from build123d import *

# Parameters (mm, degrees)
SKETCH_1_W          = 226
SKETCH_1_H          = 45
EXTRUDE_1_DEPTH     = 1
SKETCH_2_R          = 1.65
CUT_EXTRUDE_1_DEPTH = 116.222610628
CUT_EXTRUDE_2_DEPTH = 10
SKETCH_4_R          = 1.65
CUT_EXTRUDE_3_DEPTH = 116.222610628


with BuildPart() as part:
    # 草图1 → 凸台-拉伸1 (new body)
    with BuildSketch(Plane.XY):
        Rectangle(SKETCH_1_W, SKETCH_1_H)
    extrude(amount=EXTRUDE_1_DEPTH)

    # 草图2 → 切除-拉伸1 (cut, through all)
    with BuildSketch(Plane.XY.offset(1)):
        with Locations((90, 19.5)):
            Circle(SKETCH_2_R)
        with Locations((70, 19.5)):
            Circle(SKETCH_2_R)
        with Locations(Location((-70, 19.5, 0), (0, 0, 180))):
            Circle(SKETCH_2_R)
        with Locations(Location((-90, 19.5, 0), (0, 0, 180))):
            Circle(SKETCH_2_R)
    extrude(amount=-CUT_EXTRUDE_1_DEPTH, mode=Mode.SUBTRACT)

    # 草图3 → 切除-拉伸2 (cut)
    with BuildSketch(Plane.XY.offset(1)):
        with BuildLine():
            Line((-80, 6), (80, 6))
            ThreePointArc((80, 6), (86, 0), (80, -6))
            Line((80, -6), (-80, -6))
            ThreePointArc((-80, -6), (-86, 0), (-80, 6))
        make_face()
    extrude(amount=-CUT_EXTRUDE_2_DEPTH, mode=Mode.SUBTRACT)

    # 草图4 → 切除-拉伸3 (cut, through all)
    with BuildSketch(Plane.XY.offset(1)):
        with Locations((109, 7.5)):
            Circle(SKETCH_4_R)
        with Locations((109, -12.5)):
            Circle(SKETCH_4_R)
        with Locations(Location((-109, -12.5, 0), (0, 0, 180))):
            Circle(SKETCH_4_R)
        with Locations(Location((-109, 7.5, 0), (0, 0, 180))):
            Circle(SKETCH_4_R)
    extrude(amount=-CUT_EXTRUDE_3_DEPTH, mode=Mode.SUBTRACT)


solid = part.part
Could you check a few things on this model? Use its own coordinates, in mm. A direction names the side the tool comes from. Round coordinates to 2 decimals unless told otherwise and drop trailing zeros. Write each loop counter-clockwise with the first axis right and the second up, starting at its lowest first coordinate (ties: lowest second). Pieces come first, ordered by that corner, then holes. Notation, with made-up numbers: (-40, 9) - (7, 9) arc R21 ccw to (7, 34) - close; hole circle Ø8 at (10.25, -35). An arc over 180 degrees is marked (long way). Put each result on its own line as item: value. Start each with the question number.
(1) Thinking about a two-plate mould opening in Y: for faces 1 (the cylindrical face through (86, 0.1, 0.5)), 2 (the flat face through (-2, 10, 0)), which applies, released by +Y, released by -Y, zero draft, split by the parting line, or undercut?
(2) I want a section at B-B, the plane z = 0.5. Give the number of separate pieces and of enclosed holes in the cut face, plus the area to 3 significant figures.
(3) I need wall thicknesses on probe 1 along Y at (x, z) = (90, 0.7); probe 2 along X at (y, z) = (0, 0.95); probe 3 along Y at (x, z) = (45, 0.25). Which ranges of each line are inside material? Lowest first, please.
(4) I want a section at A-A, the plane y = 0. Please give me the cut outline in (x, z).
(5) For faces 3 (the flat face through (-2, 10, 1)), 4 (the cylindrical face through (-86, -0.1, 0.5)), which set-ups out of +Z, -Z, +X, -X, +Y, -Y let a thin tool reach every point of the face, with its end or its side?
(6) I want a section at C-C, the plane x = -35.5. Please give me the cut outline in (y, z), plus the area to 3 significant figures.
Here are the results:
1. face 1: undercut
1. face 2: zero draft
2. separate pieces: 1
2. enclosed holes: 9
2. area: 8,070 mm^2
3. probe 1: y = -22.5 to 17.85, 21.15 to 22.5
3. probe 2: x = -113 to -86, 86 to 113
3. probe 3: y = -22.5 to -6, 6 to 22.5
4. outline: (-113, 0) - (-86, 0) - (-86, 1) - (-113, 1) - close; (86, 0) - (113, 0) - (113, 1) - (86, 1) - close
5. face 3: +Z, +X, -X, +Y, -Y
5. face 4: +Z, -Z
6. outline: (-22.5, 0) - (-6, 0) - (-6, 1) - (-22.5, 1) - close; (6, 0) - (22.5, 0) - (22.5, 1) - (6, 1) - close
6. area: 33.0 mm^2
